```python
from build123d import *

# Parameters (mm, degrees)
EXTRUDE_1_DEPTH = 2
EXTRUDE_2_DEPTH = 8
EXTRUDE_3_DEPTH = 2
SKETCH_4_R      = 4.95
EXTRUDE_4_DEPTH = 8
EXTRUDE_5_DEPTH = 3
SKETCH_6_R      = 0.3
SKETCH_6_R_2    = 0.4
EXTRUDE_6_DEPTH = 3


with BuildPart() as part:
    # Эскиз1 → Бобышка-Вытянуть1 (new body)
    with BuildSketch(Plane.XY):
        Polygon((0, 17.9), (2.8, 17.9), (6.4, 14.342331177), (6.4, 3.557668823), (2.8, 0), (0, 0), (-3.6, 3.557668823), (-3.6, 14.342331177), align=None)
    extrude(amount=EXTRUDE_1_DEPTH)

    # Эскиз2 → Бобышка-Вытянуть2 (add)
    with BuildSketch(Plane.XY.offset(2)):
        with BuildLine():
            Line((6.4, 5.63337521), (6.4, 3.557668823))
            Line((6.4, 3.557668823), (2.8, 0))
            Line((2.8, 0), (0, 0))
            Line((0, 0), (-3.6, 3.557668823))
            Line((-3.6, 3.557668823), (-3.6, 5.63337521))
            ThreePointArc((-3.6, 5.63337521), (1.4, 2.95), (6.4, 5.63337521))
        make_face()
        with BuildLine():
            Line((-3.6, 12.26662479), (-3.6, 14.342331177))
            Line((-3.6, 14.342331177), (0, 17.9))
            Line((0, 17.9), (2.8, 17.9))
            Line((2.8, 17.9), (6.4, 14.342331177))
            Line((6.4, 14.342331177), (6.4, 12.26662479))
            ThreePointArc((6.4, 12.26662479), (1.4, 14.95), (-3.6, 12.26662479))
        make_face()
    extrude(amount=EXTRUDE_2_DEPTH)

    # Эскиз3 → Бобышка-Вытянуть3 (add)
    with BuildSketch(Plane.XY.offset(10)):
        Polygon((-3.6, 14.342331177), (-3.6, 3.557668823), (0, 0), (2.8, 0), (6.4, 3.557668823), (6.4, 14.342331177), (2.8, 17.9), (0, 17.9), align=None)
    extrude(amount=EXTRUDE_3_DEPTH)

    # Эскиз4 → Бобышка-Вытянуть4 (add)
    with BuildSketch(Plane.XY.offset(2)):
        with Locations(Location((1.4, 8.95, 0), (0, 0, 180))):
            Circle(SKETCH_4_R)
    extrude(amount=EXTRUDE_4_DEPTH)

    # Эскиз5 → Бобышка-Вытянуть5 (add)
    with BuildSketch(Plane.XY):
        with BuildLine():
            Line((9.599401359, 12.544204897), (-6.796786669, 12.544204897))
            Line((-6.796786669, 12.544204897), (-8.632281469, 10.730293057))
            ThreePointArc((-8.632281469, 10.730293057), (-9.375, 8.952102448), (-8.632281469, 7.17391184))
            Line((-8.632281469, 7.17391184), (-6.796786669, 5.36))
            Line((-6.796786669, 5.36), (9.599401359, 5.36))
            Line((9.599401359, 5.36), (11.434896159, 7.17391184))
            ThreePointArc((11.434896159, 7.17391184), (12.177614691, 8.952102448), (11.434896159, 10.730293057))
            Line((11.434896159, 10.730293057), (9.599401359, 12.544204897))
        make_face()
    extrude(amount=EXTRUDE_5_DEPTH)

    # Эскиз6 → Бобышка-Вытянуть6 (add)
    with BuildSketch(Plane.XY):
        with Locations((10.38, 8.950654336)):
            Circle(SKETCH_6_R)
        with Locations((8.584, 10.746654336)):
            Circle(SKETCH_6_R)
        with Locations((8.584, 7.156654336)):
            Circle(SKETCH_6_R)
        with Locations((-5.784, 10.746654336)):
            Circle(SKETCH_6_R)
        with Locations((-7.58, 8.950654336)):
            Circle(SKETCH_6_R)
        with Locations((-5.784, 7.156654336)):
            Circle(SKETCH_6_R)
        with Locations((1.4, 17.930654336)):
            Circle(SKETCH_6_R_2)
        with Locations((1.4, -0.029345664)):
            Circle(SKETCH_6_R_2)
    extrude(amount=-EXTRUDE_6_DEPTH)


solid = part.part
```
Read the model definition and answer for the solid it produces. Units are mm, in the model's axes. A direction names the side the tool comes from. Round coordinates to 2 decimals unless told otherwise and drop trailing zeros. Loops run counter-clockwise (first coordinate to the right, second up) from the corner with the lowest first, then second, coordinate; pieces in that order, holes last. Notation, with made-up numbers: (64.5, -30) -> (109.5, -30) arc R14 ccw to (109.5, -6) -> close; hole circle Ø9 at (76, -32.5). An arc over 180 degrees is marked (long way). One line per item, written item: value.
1) A cutting plane is placed at A-A (z = 8.25). Determine the outline of the cut face in (x, y), and give its area (3 significant figures).
Answer list:
outline: (-3.6, 3.56) -> (0, 0) -> (2.8, 0) -> (6.4, 3.56) -> (6.4, 5.63) arc R6 cw to (-3.6, 5.63) -> close; (-3.6, 12.27) arc R6 cw to (6.4, 12.27) -> (6.4, 14.34) -> (2.8, 17.9) -> (0, 17.9) -> (-3.6, 14.34) -> close; circle Ø9.9 at (1.4, 8.95)
area: 126 mm²
2) A cutting plane is placed at D-D (z = -0.5). Determine the outline of the cut face in (x, y).
Answer list:
outline: circle Ø0.6 at (-7.58, 8.95); circle Ø0.6 at (-5.78, 7.16); circle Ø0.6 at (-5.78, 10.75); circle Ø0.8 at (1.4, -0.03); circle Ø0.8 at (1.4, 17.93); circle Ø0.6 at (8.58, 7.16); circle Ø0.6 at (8.58, 10.75); circle Ø0.6 at (10.38, 8.95)
3) A cutting plane is placed at B-B (x = 1.4). Determine the outline of the cut face in (y, z), and give its area (3 significant figures).
Answer list:
outline: (-0.43, -3) -> (0.37, -3) -> (0.37, 0) -> (17.53, 0) -> (17.53, -3) -> (18.33, -3) -> (18.33, 0) -> (17.9, 0) -> (17.9, 12) -> (0, 12) -> (0, 0) -> (-0.43, 0) -> close; hole (2.95, 2) -> (4, 2) -> (4, 10) -> (2.95, 10) -> close; hole (13.9, 2) -> (14.95, 2) -> (14.95, 10) -> (13.9, 10) -> close
area: 203 mm²
4) Consider L1, parallel to Y at x = -1.5, z = 5.25; L2, parallel to Y at x = 4.75, z = 3.25; L3, parallel to Y at x = -5.75, z = -1.5. Determine where each line is inside the solid, lowest interval first. Write a range as [from, to].
Answer list:
L1: y = [1.48, 3.7], [4.94, 12.96], [14.2, 16.42]
L2: y = [1.93, 3.97], [5.31, 12.59], [13.93, 15.97]
L3: y = [6.86, 7.45], [10.45, 11.04]
5) A cutting plane is placed at C-C (x = 10.38). Determine the outline of the cut face in (y, z).
Answer list:
outline: (6.13, 0) -> (8.65, 0) -> (8.65, -3) -> (9.25, -3) -> (9.25, 0) -> (11.77, 0) -> (11.77, 3) -> (6.13, 3) -> close
6) For faces 5 (the face through (-1.825, 1.804, 5.916)), 6 (the face through (1, 17.9, 6)), 7 (the face through (5.5, 12.544, 2.5)), 8 (the face through (-5, 12.544, 1)), determine the directions among +Z, -Z, +X, -X, +Y, -Y from which every point of the face is accessible in a straight line to the end or side of a thin tool.
Answer list:
face 5: +Z, -Z, -X, -Y
face 6: +Z, +X, -X, +Y
face 7: none
face 8: +Z, -Z, -X, +Y
7) The mould has two halves that part along X. Classify faces 1 (the face through (-7.73, 6.28, 1.48)), 2 (the face through (4.57, 1.75, 5.92)), 3 (the face through (-2.7, 12.544, 2.5)), 4 (the face through (8, 5.36, 1)): pulls with the +X half, pulls with the -X half, needs draft (parallel to the pull), parting line crosses it, or undercut.
Answer list:
face 1: pulls with the -X half
face 2: pulls with the +X half
face 3: undercut
face 4: needs draft
8) Flat-ended cylindrical pins translate along their axes: P1, Ø3.5, axis at x = 8, z = 1.5, coming from the +Y side; P2, Ø1, axis at x = -4, z = 8, coming from the +Y side; P3, Ø6, axis at x = 7.5, z = 4, coming from the +Y side. Find the tip coordinate at first contact, or state that the pin passes through.
Answer list:
P1: stops at y = 14.49
P2: stops at y = 14.44
P3: stops at y = 16.22
